Model file for the job. Use its own axes, mm. Face numbers are marked on the shaded views. Coordinates: 2 decimals unless noted, no trailing zeros. Order: outer loops, then holes, each group sorted by start corner. A loop starts at its lowest first (then second) coordinate and runs counter-clockwise, first axis right, second up. Notation, with made-up numbers: (-16, 71) -> (-7, 71) arc R18 cw to (-7, 90) -> close; hole circle Ø10 at (61, 39.5). An arc over 180 degrees is marked (long way). Return JSON: item names as keys, results as strings. Group by question number.
1) Flat gauge pins, fed straight in: pin 1 (12 mm diameter, centred on x = 35.5, z = 18.5, fed in from +Y); pin 2 (2 mm diameter, centred on x = 5, z = 11.5, fed in from -Y); pin 3 (1.1 mm diameter, centred on y = 34.5, z = 6.5, fed in from +X). Where does each tip first touch, or does it go through?
2) Cut at D-D (y = 7). Write the cut outline in (x, z), and give its area (3 significant figures).
3) Cut at C-C (y = 29.5). Write the cut outline in (x, z).
4) Pull direction Y, two halves, no side cores. Call the marked faces 1, 2, 3 and 4: +Y half, -Y half, draft (parallel to the pull), parting line (faces both ways), or undercut.
5) Cut at A-A (x = 35). Write the cut outline in (y, z).
6) Probe line 1 (Z direction, x = 37.25, y = 29.5); line 2 (Y direction, x = 20, z = 15.75); line 3 (Z direction, x = 5, y = 3.5). List the from-to ranges inside material, lowest first.
7) Cut at B-B (z = 11). Write the cut outline in (x, y).
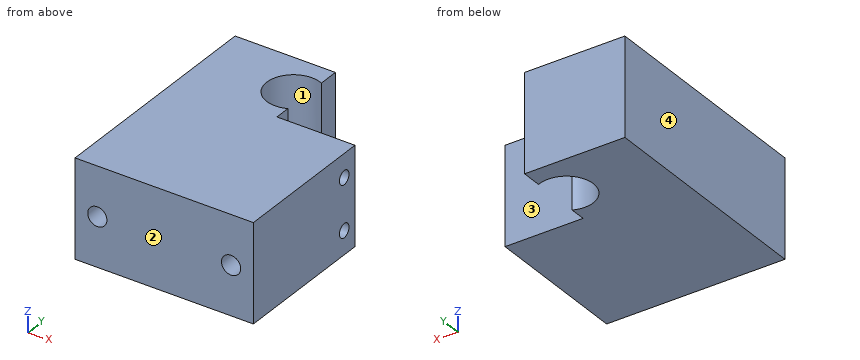
from build123d import *

# Parameters (mm, degrees)
F0_W      = 40
F0_H      = 52
F1_DEPTH  = 22
F3_R      = 6
F4_DEPTH  = 25
F5_R      = 2.15
F6_DEPTH  = 10
F7_W      = 17.5
F7_H      = 22
F8_DEPTH  = 19
F9_R      = 1.55
F10_DEPTH = 10


with BuildPart() as f1:
    # F0 (on Top) → F1 (new body)
    with BuildSketch(Plane.XY):
        with Locations((20, 26)):
            Rectangle(F0_W, F0_H)
    extrude(amount=F1_DEPTH)

    # F3 (on face) → F4 (cut)
    with BuildSketch(Plane.XY.offset(22)):
        with Locations((20, 42)):
            Circle(F3_R)
    extrude(amount=-F4_DEPTH, mode=Mode.SUBTRACT)

    # F5 (on face) → F6 (cut)
    with BuildSketch(Plane.XZ):
        with Locations((5, 11)):
            Circle(F5_R)
        with Locations((35, 11)):
            Circle(F5_R)
    extrude(amount=-F6_DEPTH, mode=Mode.SUBTRACT)

    # F7 (on face) → F8 (cut)
    with BuildSketch(Plane(origin=(0, 52, 0), x_dir=(-1, 0, 0), z_dir=(0, 1, 0))):
        with Locations((-31.25, 11)):
            Rectangle(F7_W, F7_H)
    extrude(amount=-F8_DEPTH, mode=Mode.SUBTRACT)

    # F9 (on face) → F10 (cut)
    with BuildSketch(Plane.YZ.offset(40)):
        with Locations((29.5, 16.75)):
            Circle(F9_R)
        with Locations((29.5, 5.25)):
            Circle(F9_R)
    extrude(amount=-F10_DEPTH, mode=Mode.SUBTRACT)


solid = f1.part
Answers below:
{
 "1": {"pin 1": "stops at y = 33", "pin 2": "stops at y = 10", "pin 3": "stops at x = 22.5"},
 "2": {"outline": "(0, 0) -> (40, 0) -> (40, 22) -> (0, 22) -> close; hole circle Ø4.3 at (5, 11); hole circle Ø4.3 at (35, 11)", "area": "851 mm^2"},
 "3": {"outline": "(0, 0) -> (40, 0) -> (40, 3.7) -> (30, 3.7) -> (30, 6.8) -> (40, 6.8) -> (40, 15.2) -> (30, 15.2) -> (30, 18.3) -> (40, 18.3) -> (40, 22) -> (0, 22) -> close"},
 "4": {"face 1": "undercut", "face 2": "-Y half", "face 3": "+Y half", "face 4": "draft"},
 "5": {"outline": "(0, 0) -> (33, 0) -> (33, 22) -> (0, 22) -> (0, 13.15) -> (10, 13.15) -> (10, 8.85) -> (0, 8.85) -> close; hole circle Ø3.1 at (29.5, 5.25); hole circle Ø3.1 at (29.5, 16.75)"},
 "6": {"line 1": "z = 0 to 3.7, 6.8 to 15.2, 18.3 to 22", "line 2": "y = 0 to 36, 48 to 52", "line 3": "z = 0 to 8.85, 13.15 to 22"},
 "7": {"outline": "(0, 0) -> (2.85, 0) -> (2.85, 10) -> (7.15, 10) -> (7.15, 0) -> (32.85, 0) -> (32.85, 10) -> (37.15, 10) -> (37.15, 0) -> (40, 0) -> (40, 33) -> (22.5, 33) -> (22.5, 36.55) arc R6 cw (long way) to (22.5, 47.45) -> (22.5, 52) -> (0, 52) -> close"}
}
